Verification items for the finished model (mm, model axes). A direction names the side the tool comes from. Coordinates: 2 decimals unless noted, no trailing zeros. Loops run counter-clockwise (first coordinate to the right, second up) from the corner with the lowest first, then second, coordinate; pieces in that order, holes last.
Q1. Material ranges on probe 1 along X at (y, z) = (19, -11); probe 2 along Z at (x, y) = (19, 65); probe 3 along Y at (x, z) = (0, -11.45), recorded low to high.
Q2. Sectioned sample at A-A (x = 0). Enter the section's corners in (y, z).
Q3. Sectioned sample at D-D (y = 12.7). Enter the section's corners in (x, z).
Q4. Access from +Z, -Z, +X, -X, +Y, -Y to the whole of each face (thin tool, end or side, straight path). Record for faces 1 (the face through (0, 38, 12.7)), 2 (the face through (0, 38, 11.112)).
Q5. Sectioned sample at C-C (y = 57.15). Enter the section's corners in (x, z).
Q6. Mould release check, pull along X, two halves, no side actions. Record for faces 3 (the face through (-25.4, 38, 0)), 4 (the face through (18.808, 11.484, -11.895)), 5 (the face through (0, 76.2, -12)): +X half, -X half, draft (parallel to the pull), parting line (faces both ways), or undercut.
Q7. Sectioned sample at B-B (z = 10.25). Enter the section's corners in (x, y).
Autodesk Inventor part; units mm, degrees
ref_plane "YZ Plane" through (0, 0, 0) normal (1, 0, 0) x (0, 1, 0)
ref_plane "XZ Plane" through (0, 0, 0) normal (0, 1, 0) x (-1, 0, 0)
ref_plane "XY Plane" through (0, 0, 0) normal (0, 0, 1) x (1, 0, 0)
sketch "Sketch1" plane through (0, 0, 0) normal (0, 1, 0) x (-1, 0, 0)
  line L0 (-25.4, -12.7) -> (25.4, -12.7)
  line L1 (25.4, -12.7) -> (25.4, 12.7)
  line L2 (25.4, 12.7) -> (-25.4, 12.7)
  line L3 (-25.4, 12.7) -> (-25.4, -12.7)
  line L4 (-25.4, -12.7) -> (25.4, 12.7) construction
  line L5 (25.4, -12.7) -> (-25.4, 12.7) construction
  line L6 (-23.8125, -11.9062) -> (23.8125, 11.9062) construction
  line L7 (23.8125, -11.9062) -> (-23.8125, 11.9062) construction
  line L8 (23.8125, 11.1125) -> (-23.8125, 11.1125)
  line L9 (-23.8125, 11.1125) -> (-23.8125, -11.1125)
  line L10 (-23.8125, -11.1125) -> (23.8125, -11.1125)
  line L11 (23.8125, -11.1125) -> (23.8125, 11.1125)
  point P0 (0, 0)
  dimension "d1" = 25.4
  dimension "d4" = 50.8
  dimension "d7" = 1.5875
  dimension "d8" = 1.5875
  dimension "d9" = 1.5875
  dimension "d10" = 1.5875
extrude "Extrusion2" add sketch "Sketch1" along normal blind 76.2
sketch "Sketch2" plane through (-25.4, 0, 12.7) normal (0, 0, 1) x (1, 0, 0)
  circle A0 centre (25.4, 57.15) radius 14.2875
  circle A1 centre (9.525, 12.7) radius 3.175
  circle A2 centre (41.275, 12.7) radius 3.175
  line L0 (0, 0) -> (0, 76.2)
  line L1 (0, 0) -> (50.8, 0)
  line L2 (0, 76.2) -> (50.8, 76.2)
  point P0 (25.4, 0)
  dimension "d13" = 28.575
  dimension "d14" = 31.75
  dimension "d15" = 9.525
  dimension "d16" = 12.7
  dimension "d17" = 12.7
  dimension "d18" = 19.05
  dimension "d19" = 6.35
  dimension "d20" = 6.35
extrude "Extrusion3" cut sketch "Sketch2" against normal blind 76.2
equation "\"d8\" = d7"
equation "\"d9\" = d7"
equation "\"d10\" = d7"
properties part number "1x2 hexshaft mount"
Geometry check:
1. probe 1: x = -25.4 to -23.81, 23.81 to 25.4
1. probe 2: z = -12.7 to -11.11, 11.11 to 12.7
1. probe 3: y = 0 to 42.86, 71.44 to 76.2
2. outline: (0, -12.7) - (42.86, -12.7) - (42.86, -11.11) - (0, -11.11) - close; (0, 11.11) - (42.86, 11.11) - (42.86, 12.7) - (0, 12.7) - close; (71.44, -12.7) - (76.2, -12.7) - (76.2, -11.11) - (71.44, -11.11) - close; (71.44, 11.11) - (76.2, 11.11) - (76.2, 12.7) - (71.44, 12.7) - close
3. outline: (-25.4, -12.7) - (-19.05, -12.7) - (-19.05, -11.11) - (-23.81, -11.11) - (-23.81, 11.11) - (-19.05, 11.11) - (-19.05, 12.7) - (-25.4, 12.7) - close; (-12.7, -12.7) - (12.7, -12.7) - (12.7, -11.11) - (-12.7, -11.11) - close; (-12.7, 11.11) - (12.7, 11.11) - (12.7, 12.7) - (-12.7, 12.7) - close; (19.05, -12.7) - (25.4, -12.7) - (25.4, 12.7) - (19.05, 12.7) - (19.05, 11.11) - (23.81, 11.11) - (23.81, -11.11) - (19.05, -11.11) - close
4. face 1: +Z, +X, -X, +Y, -Y
4. face 2: +Y, -Y
5. outline: (-25.4, -12.7) - (-14.29, -12.7) - (-14.29, -11.11) - (-23.81, -11.11) - (-23.81, 11.11) - (-14.29, 11.11) - (-14.29, 12.7) - (-25.4, 12.7) - close; (14.29, -12.7) - (25.4, -12.7) - (25.4, 12.7) - (14.29, 12.7) - (14.29, 11.11) - (23.81, 11.11) - (23.81, -11.11) - (14.29, -11.11) - close
6. face 3: -X half
6. face 4: undercut
6. face 5: draft
7. outline: (-25.4, 0) - (-23.81, 0) - (-23.81, 76.2) - (-25.4, 76.2) - close; (23.81, 0) - (25.4, 0) - (25.4, 76.2) - (23.81, 76.2) - close
